For this review, take the finished solid that the model builds, in its own axes (mm). A direction names the side the tool comes from. Give positions to 0.01 mm unless a question says otherwise; leave off trailing zeros. Order: outer loops, then holes, each group sorted by start corner. A loop starts at its lowest first (then second) coordinate and runs counter-clockwise, first axis right, second up. Notation, with made-up numbers: M 42,35.25 L 47,35.25 A26 ccw 47,66.25 Z; hole C 86,-22 d11. An arc over 180 degrees is marked long. Answer as CSV lines item,"result". Start each with the question number.
1. For line 1 along Z through (x, y) = (-0.7, 146.8); line 2 along Z through (x, y) = (-2.1, 146.8); line 3 along Y through (x, z) = (-1.6, 13.7), list the stretches that pass through material, from the lowest coordinate up.
2. Machinability: for faces 1 (the flat face through (-0.5, -4.8, -10.8)), 2 (the flat face through (-1, 110, 3)), which of the approach directions +Z, -Z, +X, -X, +Y, -Y give a long, thin tool a straight path to every point of the face, cutting with its end or side? Answer none if there is none.
3. We need section D-D, the plane y = 13. Give the boundary of the cut face in (x, z), and give its area (3 significant figures).
4. Clearance check with a flat-ended pin moving along its axis: P1, Ø1.5, axis at x = -2, z = 13, coming from the -Y side. State where the tip first meets the part, or that it passes through.
5. We need section C-C, the plane x = -2.15. Give the boundary of the cut face in (y, z).
6. Mouldability with a two-part tool opening along Y and no side actions: class faces 3 (the flat face through (-1, 71, 46)), 4 (the cylindrical face through (-1.479, 148.232, 34.594)), 5 (the flat face through (-2.014, -4.062, -10.104)) as pulls with the +Y half, pulls with the -Y half, needs draft (parallel to the pull), parting line crosses it, or undercut.
7. We need section A-A, the plane y = 31. Give the boundary of the cut face in (x, z).
8. We need section B-B, the plane z = 16.5. Give the boundary of the cut face in (x, y).
from build123d import *

# Parameters (mm, degrees)
SKETCH010_R     = 1.55
PAD005_DEPTH    = 3
SKETCH011_R     = 6
SKETCH011_R_2   = 4.7
SKETCH011_W     = 57
SKETCH011_H     = 22
POCKET005_DEPTH = 5
FILLET001_R     = 2
CHAMFER003_SIZE = 2


with BuildPart() as part:
    # Sketch010 (on ShapeBinder) → Pad005 (new body)
    with BuildSketch(Plane(origin=(0, 0, 0), x_dir=(0, 1, 0), z_dir=(-1, 0, 0))):
        Polygon((-6.3, -46), (151.3, -46), (151.3, 9.3), (148.3, 12.3), (-3.3, 12.3), (-6.3, 9.3), align=None)
        with Locations((-1.8, 7.8)):
            Circle(SKETCH010_R, mode=Mode.SUBTRACT)
        with Locations((-1.8, -34)):
            Circle(SKETCH010_R, mode=Mode.SUBTRACT)
        with Locations((146.8, 7.8)):
            Circle(SKETCH010_R, mode=Mode.SUBTRACT)
        with Locations((146.8, -34)):
            Circle(SKETCH010_R, mode=Mode.SUBTRACT)
    extrude(amount=PAD005_DEPTH)

    # Sketch011 (on ShapeBinder) → Pocket005 (cut)
    with BuildSketch(Plane(origin=(0, 0, 0), x_dir=(0, -1, 0), z_dir=(-1, 0, 0))):
        with Locations((-31, 13.7)):
            Circle(SKETCH011_R)
        with Locations((-13, 15)):
            Circle(SKETCH011_R_2)
        with Locations((-109.5, 14)):
            Rectangle(SKETCH011_W, SKETCH011_H)
    extrude(amount=POCKET005_DEPTH, mode=Mode.SUBTRACT)

    # Fillet001
    fillet001_edges = [part.edges().sort_by_distance(p)[0] for p in [
        (-1.5, 138, 3),
        (-1.5, 138, 25),
        (-1.5, 81, 25),
        (-1.5, 81, 3),
    ]]
    fillet(fillet001_edges, radius=FILLET001_R)

    # Chamfer003
    chamfer003_edges = [part.edges().sort_by_distance(p)[0] for p in [
        (-3, 72.5, -12.3),
        (-3, 151.3, 18.35),
        (-3, -6.3, 18.35),
        (-3, 149.8, -10.8),
        (-3, -4.8, -10.8),
    ]]
    chamfer(chamfer003_edges, length=CHAMFER003_SIZE)


solid = part.part
Result set:
1,line 1,"-12.3 to -9.35, -6.25 to 32.45, 35.55 to 46"
1,line 2,"-11.2 to -9.35, -6.25 to 32.45, 35.55 to 46"
1,line 3,"-5.7 to 8.48, 17.52 to 25, 37 to 81, 138 to 150.7"
2,face 1,"-Z, +X, -X, -Y"
2,face 2,"+X, -X"
3,outline,"M -3,-10.3 L -1,-12.3 L 0,-12.3 L 0,10.3 L -3,10.3 Z; M -3,19.7 L 0,19.7 L 0,46 L -3,46 Z"
3,area,"145 mm2"
4,P1,"y = -6.05"
5,outline,"M -5.15,-8.82 L -2.82,-11.15 L 147.82,-11.15 L 150.15,-8.82 L 150.15,46 L -5.15,46 Z; hole C -1.8,-7.8 d3.1; hole C -1.8,34 d3.1; hole C 13,15 d9.4; hole C 31,13.7 d12; hole M 81,5 A2 ccw 83,3 L 136,3 A2 ccw 138,5 L 138,23 A2 ccw 136,25 L 83,25 A2 ccw 81,23 Z; hole C 146.8,-7.8 d3.1; hole C 146.8,34 d3.1"
6,face 3,"needs draft"
6,face 4,"undercut"
6,face 5,"pulls with the -Y half"
7,outline,"M -3,-10.3 L -1,-12.3 L 0,-12.3 L 0,7.7 L -3,7.7 Z; M -3,19.7 L 0,19.7 L 0,46 L -3,46 Z"
8,outline,"M -3,-4.3 L -1,-6.3 L 0,-6.3 L 0,8.55 L -3,8.55 Z; M -3,17.45 L 0,17.45 L 0,25.69 L -3,25.69 Z; M -3,36.31 L 0,36.31 L 0,81 L -3,81 Z; M -3,138 L 0,138 L 0,151.3 L -1,151.3 L -3,149.3 Z"
